Autodesk Inventor part; units mm, degrees
ref_plane "YZ Plane" through (0, 0, 0) normal (1, 0, 0) x (0, 1, 0)
ref_plane "XZ Plane" through (0, 0, 0) normal (0, 1, 0) x (-1, 0, 0)
ref_plane "XY Plane" through (0, 0, 0) normal (0, 0, 1) x (1, 0, 0)
sketch "Sketch1" plane through (0, 0, 0) normal (0, 1, 0) x (-1, 0, 0)
  circle A0 centre (-31.75, 0) radius 11.0744
  circle A1 centre (24.765, 0) radius 9.652
  line L0 (-16.51, -6.35) -> (11.9662, -6.35)
  circle A2 centre (24.765, 0) radius 14.2875
  circle A3 centre (-31.75, 0) radius 16.51
  line L1 (-16.51, 6.35) -> (11.9662, 6.35)
  point P0 (0, 0)
  dimension "d15" = 22.1488
  dimension "d17" = 12.7
  dimension "d18" = 33.02
  dimension "d19" = 19.304
  dimension "d20" = 28.575
  dimension "d21" = 56.515
extrude "Extrusion2" add sketch "Sketch1" along normal blind 7.62
fillet "Fillet3" radius 25.4 4 edges at (-11.9662, 3.81, 6.35) (-11.9662, 3.81, -6.35) (16.51, 3.81, -6.35) (16.51, 3.81, 6.35)
draft "FaceDraft2" angle 3 pull direction (0, 1, 0) faces at (41.7415, 5.08, -13.1435) (14.1702, 2.54, 8.307) (8.391, 2.54, -6.6666) (0.8295, 2.54, 6.35) (2.6114, 2.54, -6.35) (-2.7671, 2.54, 6.4149) (-4.5723, 2.54, -6.6093) (-18.1739, 5.08, 12.6764) fixed edges at (48.26, 0, 0) (13.2365, 0, 7.9391) (13.2365, 0, -7.9391) (1.7204, 0, 6.35) (1.7204, 0, -6.35) (-8.9847, 0, 7.6534) (-8.9847, 0, -7.6534) (-39.0525, 0, 0)
chamfer "Chamfer1" distance 0.508 angle 45 6 edges at (-38.6532, 7.62, 0) (1.7204, 7.62, -5.9507) (1.7204, 7.62, 5.9507) (47.8607, 7.62, 0) (42.8244, 7.62, 0) (-15.113, 7.62, 0)
chamfer "Chamfer2" distance 0.508 angle 45 4 edges at (-39.0525, 0, 0) (1.7204, 0, -6.35) (1.7204, 0, 6.35) (48.26, 0, 0)
properties part number "Connecting Rod"
Could you check a few things on this model? Use its own coordinates, in mm. A direction names the side the tool comes from. Give positions to 0.01 mm unless a question says otherwise; leave off trailing zeros. Order: outer loops, then holes, each group sorted by start corner. A loop starts at its lowest first (then second) coordinate and runs counter-clockwise, first axis right, second up.
1. Suppose I cut it at C-C (y = 5.5). State how many separate pieces and enclosed holes the cut face has, plus the area to 3 significant figures.
Answers below:
separate pieces: 1
enclosed holes: 2
area: 1,150 mm2
2. Suppose I cut it at B-B (x = 31.75). Write out the boundary of the cut face in (y, z), plus the area to 3 significant figures.
Answers below:
outline: (0, -16) - (0.51, -16.48) - (7.11, -16.14) - (7.62, -15.6) - (7.62, -11.58) - (7.11, -11.07) - (0, -11.07) - close; (0, 11.07) - (7.11, 11.07) - (7.62, 11.58) - (7.62, 15.6) - (7.11, 16.14) - (0.51, 16.48) - (0, 16) - close
area: 79.0 mm2
3. I need wall thicknesses on L1, parallel to X at y = 4.25, z = -2.5; L2, parallel to X at y = 5.25, z = -5.5; L3, parallel to Z at x = 31.75, y = 2.25. Which ranges of each line are inside material? Lowest first, please.
Answers below:
L1: x = -38.61 to -34.09, -15.44 to 20.96, 42.54 to 47.84
L2: x = -37.65 to -32.7, -16.83 to 22.14, 41.36 to 47.02
L3: z = -16.39 to -11.07, 11.07 to 16.39
4. Thinking about a two-plate mould opening in X: for faces 1 (the cylindrical face through (42.814, 3.506, -0.487)), 2 (the flat face through (5, 7.62, 0)), which applies, +X half, -X half, draft (parallel to the pull), parting line (faces both ways), or undercut?
Answers below:
face 1: undercut
face 2: draft
5. Suppose I cut it at A-A (z = 0). Write out the boundary of the cut face in (x, y) (1 decimal), plus the area to 3 significant figures.
Answers below:
outline: (-39, 0.5) - (-38.5, 0) - (-34.4, 0) - (-34.4, 7.1) - (-34.9, 7.6) - (-38.1, 7.6) - (-38.7, 7.1) - close; (-15.1, 0) - (20.7, 0) - (20.7, 7.1) - (20.2, 7.6) - (-14.6, 7.6) - (-15.1, 7.1) - close; (42.8, 0) - (47.8, 0) - (48.2, 0.5) - (47.9, 7.1) - (47.4, 7.6) - (43.3, 7.6) - (42.8, 7.1) - close
area: 345 mm2
6. For pin 1 (10 mm diameter, centred on x = -20.5, z = 7.5, fed in from +Y); pin 2 (3 mm diameter, centred on y = 5.5, z = -9.5, fed in from -X); pin 3 (1.5 mm diameter, centred on y = 4, z = 2.5, fed in from +X), each with a flat end and sliding along its axis, tell me the tip position at first contact or that it passes through.
Answers below:
pin 1: stops at y = 7.62
pin 2: stops at x = -36.26
pin 3: stops at x = 47.97
7. Which directions (+Z, -Z, +X, -X, +Y, -Y) give clear straight access to the entire face, cutting with the end or side of a thin tool? Please do faces 3 (the flat face through (1.758, 3.764, 6.153)), 4 (the flat face through (1.758, 3.764, -6.153)), 5 (the cylindrical face through (-33.68, 3.51, 3.7)).
Answers below:
face 3: +Z, +Y
face 4: -Z, +Y
face 5: +Y, -Y
